Work out the finished part from the listing and answer in its coordinate system (mm). A direction names the side the tool comes from. Coordinates: 2 decimals unless noted, no trailing zeros. Loops run counter-clockwise (first coordinate to the right, second up) from the corner with the lowest first, then second, coordinate; pieces in that order, holes last. Notation, with made-up numbers: (41, 56) -> (89, 56) arc R23 ccw to (89, 77) -> close; hole circle Ø2 at (39, -32). An arc over 180 degrees is marked (long way). Use a Markdown table: item, result.
from build123d import *

# Parameters (mm, degrees)
SZKIC1_W                    = 4.5
SZKIC1_H                    = 37
WYTNIJ_WYCI_GNI_CIE1_DEPTH  = 9
DODANIE_WYCI_GNI_CIE1_START = 9
DODANIE_WYCI_GNI_CIE1_DEPTH = 9
SZKIC6_W                    = 1
SZKIC6_H                    = 34
SZKIC7_W                    = 0.95
SZKIC7_H                    = 3.25
OTW_R_1_9_1_9_2_D           = 1.9
SFAZOWANIE1_SIZE            = 0.3


with BuildPart() as part:
    # Szkic1 → Obrót1 (revolve)
    with BuildSketch(Plane(origin=(0, 0, 0), x_dir=(-1, 0, 0), z_dir=(0, 0, -1)), mode=Mode.PRIVATE) as obr_t1_sk:
        with Locations((-2.25, -18.5)):
            Rectangle(SZKIC1_W, SZKIC1_H)
    revolve(obr_t1_sk.sketch.rotate(Axis((0, -37, 0), (0, 1, 0)), 270), axis=Axis((0, -37, 0), (0, 1, 0)))

    # Szkic2 → Wytnij-wyciągnięcie1 (cut)
    with BuildSketch(Plane.XZ.offset(37)):
        with BuildLine():
            Line((-4.322904116, -1.25), (4.322904116, -1.25))
            ThreePointArc((4.322904116, -1.25), (0, 4.5), (-4.322904116, -1.25))
        make_face()
    extrude(amount=-WYTNIJ_WYCI_GNI_CIE1_DEPTH, mode=Mode.SUBTRACT)

    # Szkic3 → Dodanie-wyciągnięcie1 (add)
    with BuildSketch(Plane.XZ.offset(28).offset(DODANIE_WYCI_GNI_CIE1_START)):
        with BuildLine():
            Line((4.322904116, 1.25), (-4.322904116, 1.25))
            ThreePointArc((-4.322904116, 1.25), (0, 4.5), (4.322904116, 1.25))
        make_face()
    extrude(amount=-DODANIE_WYCI_GNI_CIE1_DEPTH)

    # Szkic4 → Otwór1 (revolve, cut)
    with BuildSketch(Plane(origin=(0, 0, 0), x_dir=(0, 0, 1), z_dir=(1, 0, 0))):
        Polygon((0, 0), (0, 6.5), (2.5, 6.5), (3.5, 0), align=None)
    revolve(axis=Axis((0, -110, 0), (0, 1, 0)), mode=Mode.SUBTRACT)

    # Szkic6 → Obrót2 (revolve)
    with BuildSketch(Plane(origin=(0, 0, 0), x_dir=(-1, 0, 0), z_dir=(0, 0, -1)), mode=Mode.PRIVATE) as obr_t2_sk:
        with Locations((-0.5, 10.5)):
            Rectangle(SZKIC6_W, SZKIC6_H)
    revolve(obr_t2_sk.sketch.rotate(Axis((0, -6.5, 0), (0, 1, 0)), 270), axis=Axis((0, -6.5, 0), (0, 1, 0)))

    # Szkic7 → Otwór Ø1.9 (1.9)1 (revolve, cut)
    with BuildSketch(Plane(origin=(0, -33, 1.25), x_dir=(0, 1, 0), z_dir=(1, 0, 0))):
        with Locations((0.475, 1.625)):
            Rectangle(SZKIC7_W, SZKIC7_H)
    revolve(axis=Axis((0, -33, -5.1), (0, 0, 1)), mode=Mode.SUBTRACT)

    # Otwór Ø1.9 (1.9)2 (through all)
    with Locations(Plane.XY.offset(-1.25)):
        with Locations((0, -33)):
            Hole(OTW_R_1_9_1_9_2_D / 2)

    # Sfazowanie1
    sfazowanie1_edges = [part.edges().sort_by_distance(p)[0] for p in [
        (0, -37, 4.5),
        (0, -37, -4.5),
    ]]
    chamfer(sfazowanie1_edges, length=SFAZOWANIE1_SIZE)


solid = part.part
Q1. Section C-C on y = -24.5 is taken. Determine the outline of the cut face in (x, z).
Solved:
| item | result |
|---|---|
| outline | circle Ø9 at (0, 0) |
Q2. For faces 4 (the flat face through (-1.02, -32.56, -1.25)), 5 (the cylindrical face through (-1, 11, 0)), 6 (the flat face through (0, -37, 2)), determine the directions among +Z, -Z, +X, -X, +Y, -Y from which every point of the face is accessible in a straight line to the end or side of a thin tool.
Solved:
| item | result |
|---|---|
| face 4 | +X, -X, -Y |
| face 5 | +Y |
| face 6 | +Z, -Z, +X, -X, -Y |
Q3. Given pin 1 Ø1 at (y, z) = (-14.5, -2) entering from -X; pin 2 Ø4 at (x, y) = (-0.5, 21) entering from -Z; pin 3 Ø0.8 at (x, z) = (-0.5, -0.5) entering from -Y, each flat-ended and moving along its own axis, determine where each tip first touches the part or whether it passes through.
Solved:
| item | result |
|---|---|
| pin 1 | x = -4.24 |
| pin 2 | z = -1 |
| pin 3 | y = -28 |
Q4. Section A-A on z = 0 is taken. Determine the outline of the cut face in (x, y).
Solved:
| item | result |
|---|---|
| outline | (-4.5, -28) -> (4.5, -28) -> (4.5, 0) -> (3.5, 0) -> (2.5, -6.5) -> (1, -6.5) -> (1, 27.5) -> (-1, 27.5) -> (-1, -6.5) -> (-2.5, -6.5) -> (-3.5, 0) -> (-4.5, 0) -> close |
Q5. Section B-B on y = 10.5 is taken. Determine the outline of the cut face in (x, z), and give its area (3 significant figures).
Solved:
| item | result |
|---|---|
| outline | circle Ø2 at (0, 0) |
| area | 3.14 mm² |
Q6. Consider line 1 (Z direction, x = -3.75, y = -28.5); line 2 (X direction, y = -33, z = 3.3); line 3 (Y direction, x = -0.5, z = 3.5). Determine where each line is inside the solid, lowest interval first. Write a range as [from, to].
Solved:
| item | result |
|---|---|
| line 1 | [-2.49, -1.25], [1.25, 2.49] |
| line 2 | [-3.06, -0.95], [0.95, 3.06] |
| line 3 | [-37, -33.81], [-32.19, 0] |
Q7. Determine the mould class of faces 1 (the flat face through (-1, -6.5, -1)), 2 (the conical face through (0.08, -36.89, -4.31)), 3 (the flat face through (0, -37, -2)) for opening direction X: pulls with the +X half, pulls with the -X half, needs draft (parallel to the pull), parting line crosses it, or undercut.
Solved:
| item | result |
|---|---|
| face 1 | undercut |
| face 2 | parting line crosses it |
| face 3 | needs draft |
